```python
from build123d import *

# Parameters (mm, degrees)
STOCK_HAMMERSAW_START                 = -20.066
STOCK_HAMMERSAW_MULTIBODY_1_OUTLINE_R = 2.2479
STOCK_HAMMERSAW_MULTIBODY_1_DEPTH     = 1.016
SKETCH1_W                             = 177.8
SKETCH1_H                             = 38.1
SKETCH1_W_2                           = 176.53
SKETCH1_H_2                           = 36.83
CUT_EXTRUDE1_DEPTH                    = 103.395714051
FILLET1_R                             = 2.54


# Read off the part's stored shape, not the designer's step: Stock-HammerSaw Multibody-1
with BuildPart() as part:
    # Stock-HammerSaw Multibody-1 outline → Stock-HammerSaw Multibody-1 (new body)
    with BuildSketch(Plane.XY.offset(STOCK_HAMMERSAW_START)):
        Polygon((6.35, 12.7), (43.8785, 12.7), (43.8785, 38.1), (50.2285, 38.1), (50.2285, 12.7), (88.9, 12.7), (88.9, 50.8), (-88.9, 50.8), (-88.9, 12.7), (-50.2285, 12.7), (-50.2285, 38.1), (-43.8785, 38.1), (-43.8785, 12.7), (-6.35, 12.7), (-6.35, 34.925), (6.35, 34.925), align=None)
        with Locations((-53.4035, 26.19375)):
            Circle(STOCK_HAMMERSAW_MULTIBODY_1_OUTLINE_R, mode=Mode.SUBTRACT)
        with Locations((53.4035, 26.19375)):
            Circle(STOCK_HAMMERSAW_MULTIBODY_1_OUTLINE_R, mode=Mode.SUBTRACT)
        with Locations((-53.4035, 37.30625)):
            Circle(STOCK_HAMMERSAW_MULTIBODY_1_OUTLINE_R, mode=Mode.SUBTRACT)
        with Locations((53.4035, 37.30625)):
            Circle(STOCK_HAMMERSAW_MULTIBODY_1_OUTLINE_R, mode=Mode.SUBTRACT)
    extrude(amount=STOCK_HAMMERSAW_MULTIBODY_1_DEPTH)

    # Sketch1 → Cut-Extrude1 (cut, through all)
    with BuildSketch(Plane(origin=(0, 0, -20.066), x_dir=(-1, 0, 0), z_dir=(0, 0, -1))):
        with Locations((0, 31.75)):
            Rectangle(SKETCH1_W, SKETCH1_H)
        with Locations((0, 31.75)):
            Rectangle(SKETCH1_W_2, SKETCH1_H_2, mode=Mode.SUBTRACT)
    extrude(amount=-CUT_EXTRUDE1_DEPTH, mode=Mode.SUBTRACT)

    # Fillet1
    fillet1_edges = [part.edges().sort_by_distance(p)[0] for p in [
        (-6.35, 13.335, -19.558),
        (88.265, 13.335, -19.558),
        (50.2285, 13.335, -19.558),
        (43.8785, 13.335, -19.558),
        (-50.2285, 13.335, -19.558),
        (-43.8785, 13.335, -19.558),
        (-88.265, 50.165, -19.558),
        (-88.265, 13.335, -19.558),
        (6.35, 13.335, -19.558),
        (88.265, 50.165, -19.558),
        (6.35, 34.925, -19.558),
        (-6.35, 34.925, -19.558),
        (-50.2285, 38.1, -19.558),
        (-43.8785, 38.1, -19.558),
        (50.2285, 38.1, -19.558),
        (43.8785, 38.1, -19.558),
    ]]
    fillet(fillet1_edges, radius=FILLET1_R)


solid = part.part
```
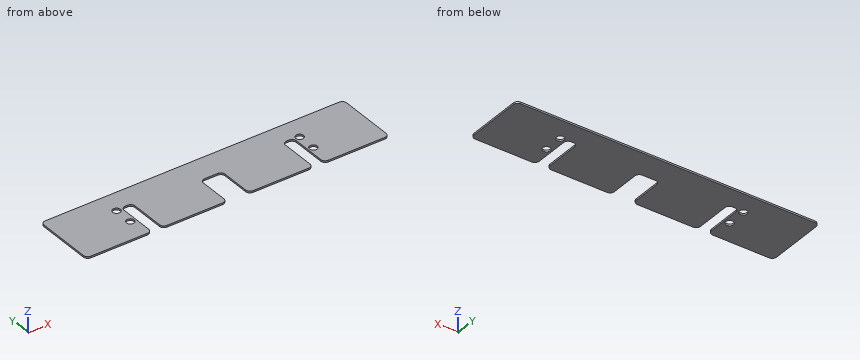
The listing builds one solid part. Answer for the finished solid, in the listing's coordinates (mm). Round coordinates to 2 decimals unless told otherwise and drop trailing zeros. Answer as CSV lines item,"result". Start each with the question number.
(1) Find the intervals of material crossed by probe 1 along X at (y, z) = (33.5, -19.35) (1 decimal); probe 2 along Y at (x, z) = (46, -19.3) (3 decimals); probe 3 along X at (y, z) = (39, -19.5) (3 decimals), in increasing order. Write a range as from..to.
(2) Flat-ended cylindrical pins translate along their axes: pin 1 Ø4 at (x, y) = (53.4, 26.19) entering from +Z; pin 2 Ø0.5 at (x, z) = (47.5, -19.5) entering from -Y. Find the tip coordinate at first contact, or state that the pin passes through.
(3) The part is cut by section A-A (y = 20). Count the separate pieces of the cut face and the enclosed holes in it, then the cut area to 3 significant figures.
Evaluation:
1,probe 1,"-88.3..-50.2, -43.9..-6.1, 6.1..43.9, 50.2..88.3"
1,probe 2,"38.065..50.165"
1,probe 3,"-88.265..-54.881, -51.926..51.926, 54.881..88.265"
2,pin 1,"through"
2,pin 2,"y = 38.1"
3,separate pieces,"4"
3,enclosed holes,"0"
3,area,"154 mm²"
